Geometry: final body of the model. Coordinates: model frame, mm. A direction names the side the tool comes from. Give positions to 0.01 mm unless a question says otherwise; leave off trailing zeros. Write each loop counter-clockwise with the first axis right and the second up, starting at its lowest first coordinate (ties: lowest second). Pieces come first, ordered by that corner, then holes. Notation, with made-up numbers: (77, 60.25) - (96, 60.25) arc R26 ccw to (96, 95.25) - close; hole circle Ø5 at (89.25, -19). An arc over 180 degrees is marked (long way). Return JSON: item names as keys, results as strings.
from build123d import *

# Parameters (mm, degrees)
F0_W     = 200
F0_H     = 100
F0_R     = 35
F1_DEPTH = 25
F2_W     = 17
F2_H     = 100
F3_DEPTH = 10


with BuildPart() as f1:
    # F0 (on Top) → F1 (new body)
    with BuildSketch(Plane.XY):
        Rectangle(F0_W, F0_H)
        Circle(F0_R, mode=Mode.SUBTRACT)
    extrude(amount=F1_DEPTH)

    # F2 (on Top) → F3 (cut)
    with BuildSketch(Plane.XY):
        with Locations((-69.6, 0)):
            Rectangle(F2_W, F2_H)
    extrude(amount=F3_DEPTH, mode=Mode.SUBTRACT)


solid = f1.part
Q1. Material intervals for probe 1 along X at (y, z) = (-41, 5.75); probe 2 along Y at (x, z) = (0, 6.5); probe 3 along X at (y, z) = (-32.5, 6), sorted ascending. Write a range as [from, to].
Answer key:
{"probe 1": "x = [-100, -78.1], [-61.1, 100]", "probe 2": "y = [-50, -35], [35, 50]", "probe 3": "x = [-100, -78.1], [-61.1, -12.99], [12.99, 100]"}
Q2. Section query C-C, the plane z = 13.25. Return the cut outline in (x, y), plus the area to 3 significant figures.
Answer key:
{"outline": "(-100, -50) - (100, -50) - (100, 50) - (-100, 50) - close; hole circle Ø70 at (0, 0)", "area": "16,200 mm^2"}
Q3. Pin query (flat end, axial travel): P1, Ø12, axis at x = -23, y = 6.5, coming from the +Z side. Return the tip coordinate at first contact, or that it passes through.
Answer key:
{"P1": "passes through"}
Q4. Section query D-D, the plane y = 41. Return the cut outline in (x, z), plus the area to 3 significant figures.
Answer key:
{"outline": "(-100, 0) - (-78.1, 0) - (-78.1, 10) - (-61.1, 10) - (-61.1, 0) - (100, 0) - (100, 25) - (-100, 25) - close", "area": "4,830 mm^2"}
Q5. Section query A-A, the plane x = 0. Return the cut outline in (y, z).
Answer key:
{"outline": "(-50, 0) - (-35, 0) - (-35, 25) - (-50, 25) - close; (35, 0) - (50, 0) - (50, 25) - (35, 25) - close"}
Q6. Section query B-B, the plane y = 0. Return the cut outline in (x, z).
Answer key:
{"outline": "(-100, 0) - (-78.1, 0) - (-78.1, 10) - (-61.1, 10) - (-61.1, 0) - (-35, 0) - (-35, 25) - (-100, 25) - close; (35, 0) - (100, 0) - (100, 25) - (35, 25) - close"}
Q7. Set-up query: faces 5 (the flat face through (-78.1, -1, 5)), 6 (the flat face through (36, 1, 0)). Return all of +Z, -Z, +X, -X, +Y, -Y with unobstructed straight access to the full face (end or side cutting, diameter ignored); none if empty.
Answer key:
{"face 5": "-Z, +Y, -Y", "face 6": "-Z, +X, -X, +Y, -Y"}
Q8. Mould query, pull axis X, two halves, no side actions, for faces 1 (the flat face through (100, -1, 12)), 2 (the flat face through (-24, -33, 25)), 3 (the flat face through (-61.1, -1, 5)), 4 (the flat face through (-100, -1, 12)). Classes: pulls with the +X half, pulls with the -X half, needs draft (parallel to the pull), parting line crosses it, or undercut.
Answer key:
{"face 1": "pulls with the +X half", "face 2": "needs draft", "face 3": "undercut", "face 4": "pulls with the -X half"}
